CAD build for the part. Positions are in the model's coordinates, mm. Face numbers are marked on the shaded views. A direction names the side the tool comes from. Round coordinates to 2 decimals unless told otherwise and drop trailing zeros. Loops run counter-clockwise (first coordinate to the right, second up) from the corner with the lowest first, then second, coordinate; pieces in that order, holes last.
from build123d import *


with BuildPart() as part:
    # Sketch1 → Revolve1 (revolve)
    with BuildSketch(Plane(origin=(0, 0, 0), x_dir=(1, 0, 0), z_dir=(0, 1, 0)), mode=Mode.PRIVATE) as revolve1_sk:
        with BuildLine():
            Line((-64.453003754, 16.1), (-53.866494762, 16.1))
            ThreePointArc((-53.866494762, 16.1), (-52.466916096, 16.1984254), (-51.094888249, 16.491764088))
            Line((-51.094888249, 16.491764088), (-40.81111926, 19.458235912))
            ThreePointArc((-40.81111926, 19.458235912), (-39.439091413, 19.7515746), (-38.039512747, 19.85))
            Line((-38.039512747, 19.85), (3.846996246, 19.85))
            Line((3.846996246, 19.85), (3.846996246, 21.35))
            Line((3.846996246, 21.35), (-38.039512747, 21.35))
            ThreePointArc((-38.039512747, 21.35), (-39.439091413, 21.2515746), (-40.81111926, 20.958235912))
            Line((-40.81111926, 20.958235912), (-51.094888249, 17.991764088))
            ThreePointArc((-51.094888249, 17.991764088), (-52.466916096, 17.6984254), (-53.866494762, 17.6))
            Line((-53.866494762, 17.6), (-64.453003754, 17.6))
            Line((-64.453003754, 17.6), (-64.453003754, 16.1))
        make_face()
    revolve(revolve1_sk.sketch.rotate(Axis((-73.729430683, 0, 0), (1, 0, 0)), 180), axis=Axis((-73.729430683, 0, 0), (1, 0, 0)))


solid = part.part
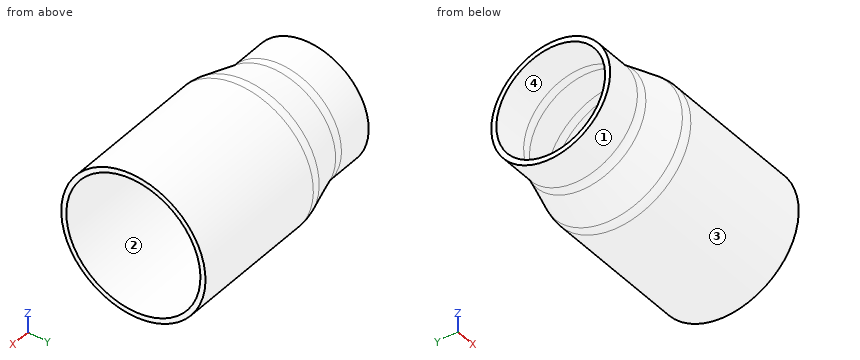
Item 1: Cut at B-B (x = -46.5). List the corners of the cut face in (y, z).
Verdict:
outline: circle Ø38.63 at (0, 0); hole circle Ø35.63 at (0, 0)
Item 2: Mould opens along Y. For the marked faces 3 and 4 say: released by +Y, released by -Y, zero draft, split by the parting line, or undercut.
Verdict:
face 3: split by the parting line
face 4: undercut
Item 3: 3-axis set-ups, long thin cutter, end or side, ignore diameter. For the marked faces 1 and 2: which of +Z, -Z, +X, -X, +Y, -Y reach the whole face in a straight line?
Verdict:
face 1: -X
face 2: +X
Item 4: Cut at A-A (x = -28). List the corners of the cut face in (y, z), plus the area to 3 significant figures.
Verdict:
outline: circle Ø42.7 at (0, 0); hole circle Ø39.7 at (0, 0)
area: 194 mm2
Item 5: Flat gauge pins, fed straight in: P1, Ø1.5, axis at x = -41.5, z = -6, coming from the +Y side; P2, Ø12, axis at x = -24.5, z = 2.5, coming from the -Y side; P3, Ø12, axis at x = -52.5, z = -0.5, coming from the +Y side. Where does each tip first touch, or does it go through?
Verdict:
P1: stops at y = 20.18
P2: stops at y = -21.35
P3: stops at y = 19.31
Item 6: Wall check: L1, parallel to Y at x = -11, z = 0; L2, parallel to Y at x = -59.5, z = 0; L3, parallel to Z at x = -49, y = -15.5. Give the ranges that are in metal, low to high.
Verdict:
L1: y = -21.35 to -19.85, 19.85 to 21.35
L2: y = -17.6 to -16.1, 16.1 to 17.6
L3: z = -10.27 to -7.21, 7.21 to 10.27
